Autodesk Inventor part; units mm, degrees
ref_plane "YZ Plane" through (0, 0, 0) normal (1, 0, 0) x (0, 1, 0)
ref_plane "XZ Plane" through (0, 0, 0) normal (0, 1, 0) x (-1, 0, 0)
ref_plane "XY Plane" through (0, 0, 0) normal (0, 0, 1) x (1, 0, 0)
sketch "Sketch1" plane through (0, 0, 0) normal (0, 0, 1) x (1, 0, 0)
  line L0 (-30, -20) -> (30, -20)
  line L1 (30, -20) -> (30, 20)
  line L2 (30, 20) -> (-30, 20)
  line L3 (-30, 20) -> (-30, -20)
  line L4 (-30, -20) -> (30, 20) construction
  line L5 (30, -20) -> (-30, 20) construction
  circle A0 centre (-27.9, 17.9) radius 2.1 construction
  circle A1 centre (-27.9, 17.9) radius 1
  line L6 (0, 0) -> (-34.17, 0) construction
  line L7 (0, 33.0444) -> (0, 0) construction
  circle A2 centre (-27.9, -17.9) radius 1
  circle A3 centre (27.9, 17.9) radius 1
  circle A4 centre (27.9, -17.9) radius 1
  line L8 (-25.8, -20) -> (-25.8, 20)
  line L9 (25.8, -20) -> (25.8, 20)
  line L10 (-27.9, 17.9) -> (27.9, 17.9)
  line L11 (27.9, -17.9) -> (-27.9, -17.9)
  circle A5 centre (-14.4721, 12.2361) radius 2.75
  circle A6 centre (-14.4721, 12.2361) radius 4.5
  circle A7 centre (-14.4721, 12.2361) radius 5 construction
  circle A8 centre (-10, 10) radius 2.5 construction
  line L12 (-34.3347, 5) -> (2.7365, 5) construction
  line L13 (-14.4721, 12.2361) -> (0, 5) construction
  circle A9 centre (-14.4721, -2.2361) radius 2.75
  circle A10 centre (-14.4721, -2.2361) radius 4.5
  circle A11 centre (14.4721, 12.2361) radius 2.75
  circle A12 centre (14.4721, 12.2361) radius 4.5
  circle A13 centre (14.4721, -2.2361) radius 2.75
  circle A14 centre (14.4721, -2.2361) radius 4.5
  line L14 (-30, -10) -> (30, -10)
  arc A15 (-17.9, -10) -> (-25.8, -17.9) centre (-17.9, -17.9) ccw
  arc A16 (25.8, -17.9) -> (17.9, -10) centre (17.9, -17.9) ccw
  point P0 (-25.8, 17.9)
  point P1 (25.8, 17.9)
  point P2 (25.8, 20)
  dimension "d0" = 60
  dimension "d1" = 40
  dimension "d2" = 1.1
  dimension "d3" = 2
  dimension "d8" = 9
  dimension "d9" = 5.5
  dimension "d10" = 10
  dimension "d20" = 5
  dimension "d22" = 5
  dimension "d25" = 10
  dimension "d26" = 10
  dimension "d27" = 5
extrude "Extrusion2" add sketch "Sketch1" along normal blind 2.5 contours L3 L14 L8 L0 | L3 L2 L8 L14 | L9 L14 L1 L0 | L14 L9 L2 L1
extrude "Extrusion3" add sketch "Sketch1" against normal blind 2.5 contours L3 L14 L8 L0 | L3 L2 L8 L14 | L9 L14 L1 L0 | L8 L14 A15 | L8 L10 L9 L14 | A16 L14 L9 | L2 L9 L10 L8 | L14 L9 L2 L1 | A6 | A10 | A12 | A14
extrude "Extrusion4" cut sketch "Sketch1" along normal blind 2.5 and the other way blind 1 contours A5 | A6 | A9 | A10 | A11 | A12 | A13 | A14
fillet "Fillet1" radius 2.1 8 edges at (-30, -20, 0) (-30, 20, 0) (30, -20, 0) (30, 20, 0) (-25.8, -20, 0) (-25.8, 20, 1.25) (25.8, 20, 1.25) (25.8, -20, 0)
properties part number "pcb"
The model under review builds one solid part; all positions refer to its coordinate system, in mm. A direction names the side the tool comes from. Coordinates: 2 decimals unless noted, no trailing zeros. Order: outer loops, then holes, each group sorted by start corner. A loop starts at its lowest first (then second) coordinate and runs counter-clockwise, first axis right, second up. Notation, with made-up numbers: (67.25, -13) -> (116.25, -13) arc R19 ccw to (116.25, 6) -> close; hole circle Ø10 at (-14.5, 57). An arc over 180 degrees is marked (long way). Answer in a Markdown table with one row per item.
(1) Wall thickness on line 1 along Y through (x, z) = (27.9, -0.1); line 2 along X through (y, z) = (-2, 1.15); line 3 along X through (y, z) = (12.5, -1.35): over which ranges is each line inside the solid? List them lowest first.
Answers:
| item | result |
|---|---|
| line 1 | -20 to -18.9, -16.9 to 16.9, 18.9 to 20 |
| line 2 | -30 to -25.8, 25.8 to 30 |
| line 3 | -30 to -17.21, -11.73 to 11.73, 17.21 to 30 |
(2) Consider section B-B (x = 16). Write out the cut boundary in (y, z), plus the area to 3 significant figures.
Answers:
| item | result |
|---|---|
| outline | (-10, -2.5) -> (-4.52, -2.5) -> (-4.52, -1) -> (-6.47, -1) -> (-6.47, 0) -> (-10, 0) -> close; (0.05, -2.5) -> (9.95, -2.5) -> (9.95, -1) -> (8, -1) -> (8, 0) -> (2, 0) -> (2, -1) -> (0.05, -1) -> close; (14.52, -2.5) -> (20, -2.5) -> (20, 0) -> (16.47, 0) -> (16.47, -1) -> (14.52, -1) -> close |
| area | 44.4 mm² |
(3) The part is to be moulded in two halves that separate along Y. For faces 4 (the cylindrical face through (-12.4, -6.23, -0.49)), 5 (the cylindrical face through (-29.4, -19.37, 0.04)), 6 (the flat face through (-28, 0, 2.5)), say which applies: +Y half, -Y half, draft (parallel to the pull), parting line (faces both ways), or undercut.
Answers:
| item | result |
|---|---|
| face 4 | undercut |
| face 5 | -Y half |
| face 6 | draft |
(4) Consider section D-D (y = -9). Write out the cut boundary in (x, z), plus the area to 3 significant figures.
Answers:
| item | result |
|---|---|
| outline | (-30, -2.5) -> (30, -2.5) -> (30, 2.5) -> (25.8, 2.5) -> (25.8, 0) -> (-25.8, 0) -> (-25.8, 2.5) -> (-30, 2.5) -> close |
| area | 171 mm² |
(5) Insertion check: pin 1 (2 mm diameter, centred on x = -1, y = 11.5, fed in from +Z); pin 2 (1.6 mm diameter, centred on x = 27.9, y = 17.9, fed in from +Z); pin 3 (7 mm diameter, centred on x = -14.47, y = -2.24, fed in from +Z). Each pin has a flat end and moves straight along its axis. Give the tip position at first contact, or say it passes through.
Answers:
| item | result |
|---|---|
| pin 1 | z = 0 |
| pin 2 | through |
| pin 3 | z = -1 |
(6) Consider section A-A (z = 1.2). State how many separate pieces and enclosed holes the cut face has, plus the area to 3 significant figures.
Answers:
| item | result |
|---|---|
| separate pieces | 2 |
| enclosed holes | 4 |
| area | 316 mm² |
(7) Machinability: for faces 1 (the cylindrical face through (-17.22, -2.12, -1.74)), 2 (the cylindrical face through (10.9, 9.5, -0.5)), 3 (the flat face through (0, -10, -1)), which of the approach directions +Z, -Z, +X, -X, +Y, -Y give a long, thin tool a straight path to every point of the face, cutting with its end or side? Answer none if there is none.
Answers:
| item | result |
|---|---|
| face 1 | +Z, -Z |
| face 2 | +Z |
| face 3 | +Z, -Z, -Y |
(8) Consider section C-C (y = -1.5). Write out the cut boundary in (x, z).
Answers:
| item | result |
|---|---|
| outline | (-30, -2.5) -> (-17.12, -2.5) -> (-17.12, -1) -> (-18.91, -1) -> (-18.91, 0) -> (-25.8, 0) -> (-25.8, 2.5) -> (-30, 2.5) -> close; (-11.82, -2.5) -> (11.82, -2.5) -> (11.82, -1) -> (10.03, -1) -> (10.03, 0) -> (-10.03, 0) -> (-10.03, -1) -> (-11.82, -1) -> close; (17.12, -2.5) -> (30, -2.5) -> (30, 2.5) -> (25.8, 2.5) -> (25.8, 0) -> (18.91, 0) -> (18.91, -1) -> (17.12, -1) -> close |
